Read the model definition and answer for the solid it produces. Units are mm, in the model's axes. A direction names the side the tool comes from. Coordinates: 2 decimals unless noted, no trailing zeros. Loops run counter-clockwise (first coordinate to the right, second up) from the corner with the lowest first, then second, coordinate; pieces in that order, holes last.
from build123d import *

# Parameters (mm, degrees)
SKETCH2_W           = 20
SKETCH2_H           = 20
BOSS_EXTRUDE1_DEPTH = 10
SKETCH5_R           = 4
BOSS_EXTRUDE2_DEPTH = 10
SKETCH3_R           = 4
BOSS_EXTRUDE3_DEPTH = 10
BOSS_EXTRUDE4_START = 10
SKETCH6_R           = 4
BOSS_EXTRUDE4_DEPTH = 10
BOSS_EXTRUDE5_START = 10
SKETCH4_R           = 4
BOSS_EXTRUDE5_DEPTH = 10


with BuildPart() as part:
    # Sketch2 → Boss-Extrude1 (new, symmetric)
    with BuildSketch(Plane(origin=(0, 0, 0), x_dir=(1, 0, 0), z_dir=(0, 1, 0))):
        Rectangle(SKETCH2_W, SKETCH2_H)
    extrude(amount=BOSS_EXTRUDE1_DEPTH, both=True)

    # Sketch5 → Boss-Extrude2 (add)
    with BuildSketch(Plane(origin=(0, 0, -10), x_dir=(-1, 0, 0), z_dir=(0, 0, -1))):
        Circle(SKETCH5_R)
    extrude(amount=BOSS_EXTRUDE2_DEPTH)

    # Sketch3 → Boss-Extrude3 (add)
    with BuildSketch(Plane(origin=(0, 10, 0), x_dir=(1, 0, 0), z_dir=(0, 1, 0))):
        with Locations(Location((0, 0, 0), (0, 0, 270))):
            Circle(SKETCH3_R)
    extrude(amount=BOSS_EXTRUDE3_DEPTH)

    # Sketch6 → Boss-Extrude4 (add)
    with BuildSketch(Plane.XY.offset(10).offset(BOSS_EXTRUDE4_START)):
        with Locations(Location((0, 0, 0), (0, 0, 180))):
            Circle(SKETCH6_R)
    extrude(amount=-BOSS_EXTRUDE4_DEPTH)

    # Sketch4 → Boss-Extrude5 (add)
    with BuildSketch(Plane.XZ.offset(10).offset(BOSS_EXTRUDE5_START)):
        with Locations(Location((0, 0, 0), (0, 0, 90))):
            Circle(SKETCH4_R)
    extrude(amount=-BOSS_EXTRUDE5_DEPTH)


solid = part.part
Q1. Flat-ended cylindrical pins translate along their axes: pin 1 Ø1 at (x, y) = (-6, 1.5) entering from +Z; pin 2 Ø1.5 at (y, z) = (-12, 1) entering from -X; pin 3 Ø10 at (x, z) = (2.5, 10.5) entering from -Y. Find the tip coordinate at first contact, or state that the pin passes through.
Findings below:
pin 1: stops at z = 10
pin 2: stops at x = -3.99
pin 3: stops at y = -10
Q2. A cutting plane is placed at A-A (x = 0). Give the vertices of the cut face in (y, z), then the cut area to 3 significant figures.
Findings below:
outline: (-20, -4) - (-10, -4) - (-10, -10) - (-4, -10) - (-4, -20) - (4, -20) - (4, -10) - (10, -10) - (10, -4) - (20, -4) - (20, 4) - (10, 4) - (10, 10) - (4, 10) - (4, 20) - (-4, 20) - (-4, 10) - (-10, 10) - (-10, 4) - (-20, 4) - close
area: 720 mm2
Q3. Straight lines are drawn through the part: probe 1 along Y at (x, z) = (-6, 9); probe 2 along Z at (x, y) = (-0.25, 17.5). For each, find the intervals that lie inside material, in ascending order.
Findings below:
probe 1: y = -10 to 10
probe 2: z = -3.99 to 3.99
Q4. A cutting plane is placed at D-D (x = 6). Give the vertices of the cut face in (y, z), then the cut area to 3 significant figures.
Findings below:
outline: (-10, -10) - (10, -10) - (10, 10) - (-10, 10) - close
area: 400 mm2
Q5. A cutting plane is placed at B-B (y = 0). Give the vertices of the cut face in (x, z).
Findings below:
outline: (-10, -10) - (-4, -10) - (-4, -20) - (4, -20) - (4, -10) - (10, -10) - (10, 10) - (4, 10) - (4, 20) - (-4, 20) - (-4, 10) - (-10, 10) - close
Q6. Which of the six approach directions +Z, -Z, +X, -X, +Y, -Y give full straight-line access (tool end or side, diameter ignored) to faces 1 (the face through (0.867, 3.905, 15.07)), 2 (the face through (0.867, -3.905, -14.93)), 3 (the face through (4.3, 10, -0.1))?
Findings below:
face 1: +Z
face 2: -Z
face 3: +Y
